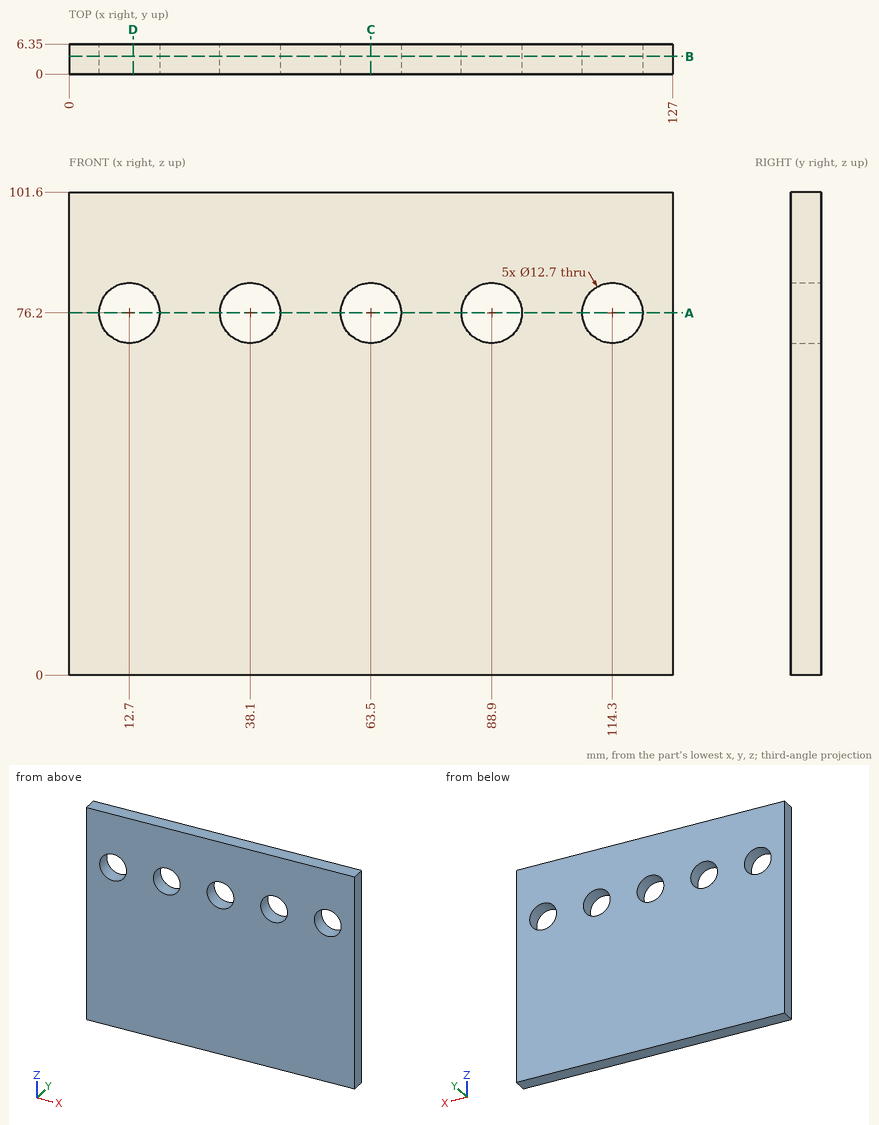
Can you work these out from the drawing? Everything is in mm from the part's minimum corner. Round coordinates to 2 decimals unless told otherwise and drop trailing zeros. Order: outer loops, then holes, each group sorted by start corner. A loop starts at its lowest first (then second) coordinate and runs counter-clockwise, first axis right, second up. Notation, with made-up numbers: M -32.5,51 L -4.5,51 A26 ccw -4.5,88 Z; hole C 47.25,85.5 d5. An arc over 180 degrees is marked long. Answer as CSV lines item,"result".
Item 1: Imagine slicing it at C-C on x = 63.5. List the corners of the cut face in (y, z) for me.
From the geometry:
outline,"M 0,0 L 6.35,0 L 6.35,69.85 L 0,69.85 Z; M 0,82.55 L 6.35,82.55 L 6.35,101.6 L 0,101.6 Z"
Item 2: Please list where these lines run through material, in increasing order: L1, parallel to X at y = 5.25, z = 76.2; L2, parallel to Z at x = 38.1, y = 4; L3, parallel to Z at x = 113, y = 2.5. Write a range as [from, to].
From the geometry:
L1,"[0, 6.35], [19.05, 31.75], [44.45, 57.15], [69.85, 82.55], [95.25, 107.95], [120.65, 127]"
L2,"[0, 69.85], [82.55, 101.6]"
L3,"[0, 69.98], [82.42, 101.6]"
Item 3: Imagine slicing it at D-D on x = 13.5. List the corners of the cut face in (y, z) for me, and give its area (3 significant figures).
From the geometry:
outline,"M 0,0 L 6.35,0 L 6.35,69.9 L 0,69.9 Z; M 0,82.5 L 6.35,82.5 L 6.35,101.6 L 0,101.6 Z"
area,"565 mm2"
Item 4: Imagine slicing it at B-B on y = 3.75. List the corners of the cut face in (x, z) for me.
From the geometry:
outline,"M 0,0 L 127,0 L 127,101.6 L 0,101.6 Z; hole C 12.7,76.2 d12.7; hole C 38.1,76.2 d12.7; hole C 63.5,76.2 d12.7; hole C 88.9,76.2 d12.7; hole C 114.3,76.2 d12.7"
Item 5: Imagine slicing it at A-A on z = 76.2. List the corners of the cut face in (x, y) for me, and give its area (3 significant figures).
From the geometry:
outline,"M 0,0 L 6.35,0 L 6.35,6.35 L 0,6.35 Z; M 19.05,0 L 31.75,0 L 31.75,6.35 L 19.05,6.35 Z; M 44.45,0 L 57.15,0 L 57.15,6.35 L 44.45,6.35 Z; M 69.85,0 L 82.55,0 L 82.55,6.35 L 69.85,6.35 Z; M 95.25,0 L 107.95,0 L 107.95,6.35 L 95.25,6.35 Z; M 120.65,0 L 127,0 L 127,6.35 L 120.65,6.35 Z"
area,"403 mm2"
